Answer from the drawing. Dimensions are ordinates in mm from the lowest x, y and z of the part. A direction names the side the tool comes from. Coordinates: 2 decimals unless noted, no trailing zeros. Write each loop counter-clockwise with the first axis right and the second up, starting at its lowest first coordinate (ties: lowest second). Pieces come first, ordered by that corner, then holes.
(1) Given pin 1 (4 mm diameter, centred on y = 25, z = 40, fed in from +X); pin 2 (1.5 mm diameter, centred on x = 9.5, y = 14.5, fed in from -Z); pin 3 (15 mm diameter, centred on x = 39.5, y = 25, fed in from +Z), each flat-ended and moving along its own axis, determine where each tip first touches the part or whether it passes through.
(2) Straight lines are drawn through the part: line 1 along X through (y, z) = (17, 23); line 2 along Z through (x, y) = (23.5, 25.5); line 3 along Y through (x, z) = (34.6, 27.5). For each, find the intervals that lie inside material, in ascending order.
(3) The part is cut by section B-B, the plane z = 36. Determine the outline of the cut face in (x, y).
(4) The part is cut by section C-C, the plane x = 34.6. Determine the outline of the cut face in (y, z).
(5) The part is cut by section D-D, the plane y = 7. Determine the outline of the cut face in (x, z).
(6) Determine the mould class of the marked faces 5, 6 and 7 for opening direction Y: pulls with the +Y half, pulls with the -Y half, needs draft (parallel to the pull), parting line crosses it, or undercut.
(7) Which of the six approach directions +Z, -Z, +X, -X, +Y, -Y give full straight-line access (tool end or side, diameter ignored) to the marked faces 1, 2, 3 and 4?
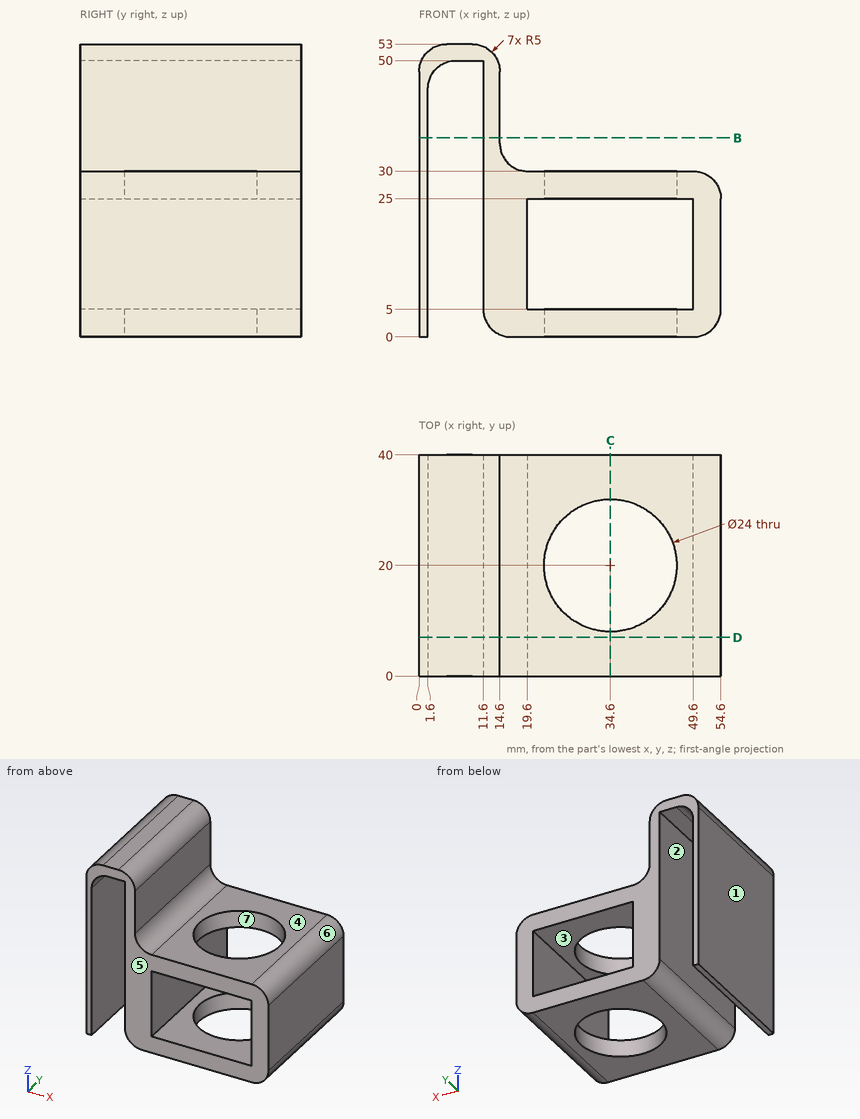
Computed:
1. pin 1: stops at x = 14.6
1. pin 2: stops at z = 50
1. pin 3: stops at z = 30
2. line 1: x = 0 to 1.6, 11.6 to 19.6, 49.6 to 54.6
2. line 2: z = 0 to 5, 25 to 30
2. line 3: y = 0 to 8, 32 to 40
3. outline: (0, 0) - (1.6, 0) - (1.6, 40) - (0, 40) - close; (11.6, 0) - (14.6, 0) - (14.6, 40) - (11.6, 40) - close
4. outline: (0, 0) - (8, 0) - (8, 5) - (0, 5) - close; (0, 25) - (8, 25) - (8, 30) - (0, 30) - close; (32, 0) - (40, 0) - (40, 5) - (32, 5) - close; (32, 25) - (40, 25) - (40, 30) - (32, 30) - close
5. outline: (0, 0) - (1.6, 0) - (1.6, 45) arc R5 cw to (6.6, 50) - (11.6, 50) - (11.6, 5) arc R5 ccw to (16.6, 0) - (49.6, 0) arc R5 ccw to (54.6, 5) - (54.6, 25) arc R5 ccw to (49.6, 30) - (19.6, 30) arc R5 cw to (14.6, 35) - (14.6, 48) arc R5 ccw to (9.6, 53) - (5, 53) arc R5 ccw to (0, 48) - close; hole (19.6, 5) - (49.6, 5) - (49.6, 25) - (19.6, 25) - close
6. face 5: pulls with the -Y half
6. face 6: needs draft
6. face 7: undercut
7. face 1: +Z, -Z, -X, +Y, -Y
7. face 2: -Z, +Y, -Y
7. face 3: +Y, -Y
7. face 4: +Z, +X, +Y, -Y
